Can you work these out from the drawing? Everything is in mm from the part's minimum corner. A direction names the side the tool comes from. Give positions to 0.01 mm unless a question says otherwise; leave off trailing zeros. Loops run counter-clockwise (first coordinate to the right, second up) from the corner with the lowest first, then second, coordinate; pieces in that order, holes last. Notation, with made-up numbers: (28, 19.5) - (37, 19.5) arc R18 cw to (37, 40.5) - close; hole circle Ø4 at (-23, 66.25). An arc over 180 degrees is marked (long way). Answer in a Markdown table with one row per item.
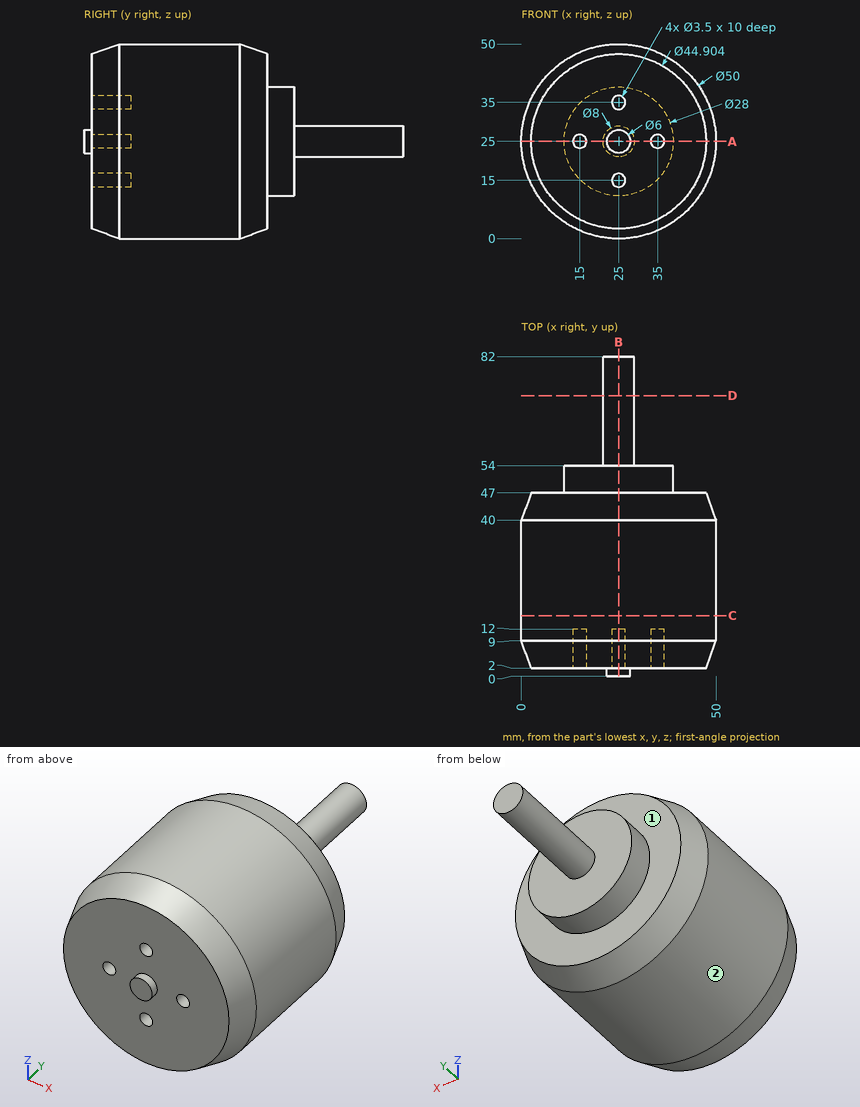
Q1. Imagine slicing it at C-C, the plane y = 15.5. Write out the boundary of the cut face in (x, z), and give its area (3 significant figures).
Checked values:
| item | result |
|---|---|
| outline | circle Ø50 at (25, 25) |
| area | 1,960 mm² |
Q2. Imagine slicing it at B-B, the plane x = 25. Write out the boundary of the cut face in (y, z).
Checked values:
| item | result |
|---|---|
| outline | (0, 22) - (2, 22) - (2, 16.75) - (12, 16.75) - (12, 13.25) - (2, 13.25) - (2, 2.55) - (9, 0) - (40, 0) - (47, 2.55) - (47, 11) - (54, 11) - (54, 21) - (82, 21) - (82, 29) - (54, 29) - (54, 39) - (47, 39) - (47, 47.45) - (40, 50) - (9, 50) - (2, 47.45) - (2, 36.75) - (12, 36.75) - (12, 33.25) - (2, 33.25) - (2, 28) - (0, 28) - close |
Q3. If I drill on line 1 (Y direction, x = 24, z = 5); line 2 (Y direction, x = 14, z = 33); line 3 (X direction, y = 10, z = 24) (1 decimal), over which ranges is the centre line in solid material (lowest first)? Write a range as [from, to].
Checked values:
| item | result |
|---|---|
| line 1 | y = [2, 47] |
| line 2 | y = [2, 54] |
| line 3 | x = [0, 13.6], [16.4, 33.6], [36.4, 50] |
Q4. Imagine slicing it at D-D, the plane y = 72. Write out the boundary of the cut face in (x, z).
Checked values:
| item | result |
|---|---|
| outline | circle Ø8 at (25, 25) |
Q5. Imagine slicing it at A-A, the plane z = 25. Write out the boundary of the cut face in (x, y), and give its area (3 significant figures).
Checked values:
| item | result |
|---|---|
| outline | (0, 9) - (2.55, 2) - (13.25, 2) - (13.25, 12) - (16.75, 12) - (16.75, 2) - (22, 2) - (22, 0) - (28, 0) - (28, 2) - (33.25, 2) - (33.25, 12) - (36.75, 12) - (36.75, 2) - (47.45, 2) - (50, 9) - (50, 40) - (47.45, 47) - (39, 47) - (39, 54) - (29, 54) - (29, 82) - (21, 82) - (21, 54) - (11, 54) - (11, 47) - (2.55, 47) - (0, 40) - close |
| area | 2,580 mm² |
Q6. For pin 1 (3 mm diameter, centred on x = 25, z = 35, fed in from -Y); pin 2 (1.5 mm diameter, centred on x = 33.5, z = 14.5, fed in from -Y); pin 3 (12 mm diameter, centred on x = 33.5, y = 63, fed in from +Z), each with a flat end and sliding along its axis, tell me the tip position at first contact or that it passes through.
Checked values:
| item | result |
|---|---|
| pin 1 | stops at y = 12 |
| pin 2 | stops at y = 2 |
| pin 3 | stops at z = 28.12 |
Q7. On a 3-axis mill with a long thin cutter (end or side, diameter ignored), from which of +Z, -Z, +X, -X, +Y, -Y can I reach the whole of each face in a straight line? I mean the marked faces 1 and 2. Say none if no direction works.
Checked values:
| item | result |
|---|---|
| face 1 | +Y |
| face 2 | +Y, -Y |
